Source: CAD feature listing. Evaluate the final solid. Frame: model axes, mm. A direction names the side the tool comes from. Give positions to 0.01 mm unless a question says otherwise; leave off trailing zeros. Order: outer loops, then holes, each group sorted by start corner. A loop starts at its lowest first (then second) coordinate and runs counter-clockwise, first axis right, second up.
1) Access query for faces 1 (the face through (2, -5, -2)), 2 (the face through (-2.003, 19.154, 0.631)), 3 (the face through (1.014, -3.768, 1.724)). Directions: +Z, -Z, +X, -X, +Y, -Y. A direction counts if a zero-diameter tool reaches every point of the face in a straight line with its end or side. Return the directions, or none.
2) Section A-A, the plane z = 0. Return loops of the section in (x, y).
3) Section B-B, the plane y = 10. Return loops of the section in (x, z), plus the area to 3 significant figures.
4) First-contact query: P1, Ø4, axis at x = -1.5, y = 1.5, coming from the -Z side; P2, Ø4, axis at y = 18.5, z = 1.5, coming from the -X side. Flat tips, straight axial feed; report the tip coordinate or a pass-through.
5) Draft query along Z for faces 4 (the face through (-2, -4, 0)), 5 (the face through (2.285, -2.268, 3.584)), 6 (the face through (0.99, -3.77, -1.74)), 7 (the face through (0, 30, 0)). Return one class per face: released by +Z, released by -Z, zero draft, split by the parting line, or undercut.
6) Material intervals for line 1 (Y direction, x = 2.5, z = -0.5); line 2 (Z direction, x = -1.5, y = 7), sorted ascending.
```python
from build123d import *

# Parameters (mm, degrees)
F0_R     = 4.25
F1_DEPTH = 5
F2_R     = 2.5
F3_DEPTH = 30
F4_R     = 2.5
F4_R_2   = 2.1
F5_DEPTH = 22
F7_DEPTH = 2.5
F8_SIZE  = 0.4


with BuildPart() as f1:
    # F0 (on Front) → F1 (new body)
    with BuildSketch(Plane.XZ):
        Circle(F0_R)
    extrude(amount=F1_DEPTH)

    # F2 (on face) → F3 (join)
    with BuildSketch(Plane(origin=(0, 0, 0), x_dir=(-1, 0, 0), z_dir=(0, 1, 0))):
        Circle(F2_R)
    extrude(amount=F3_DEPTH)

    # F4 (on face) → F5 (cut)
    with BuildSketch(Plane(origin=(0, 30, 0), x_dir=(-1, 0, 0), z_dir=(0, 1, 0))):
        Circle(F4_R)
        Circle(F4_R_2, mode=Mode.SUBTRACT)
    extrude(amount=-F5_DEPTH, mode=Mode.SUBTRACT)

    # F6 (on face) → F7 (cut)
    with BuildSketch(Plane.XZ.offset(5)):
        Polygon((0, -2.309401), (2, -1.154701), (2, 1.154701), (0, 2.309401), (-2, 1.154701), (-2, -1.154701), align=None)
    extrude(amount=-F7_DEPTH, mode=Mode.SUBTRACT)

    # F8
    f8_edges = [f1.edges().sort_by_distance(p)[0] for p in [
        (-4.25, -5, 0),
    ]]
    chamfer(f8_edges, length=F8_SIZE)


solid = f1.part
```
From the geometry:
1. face 1: +Z, -Z, +X, -X, -Y
1. face 2: +Y
1. face 3: -Y
2. outline: (-4.25, -4.6) - (-3.85, -5) - (-2, -5) - (-2, -2.5) - (2, -2.5) - (2, -5) - (3.85, -5) - (4.25, -4.6) - (4.25, 0) - (2.5, 0) - (2.5, 8) - (2.1, 8) - (2.1, 30) - (-2.1, 30) - (-2.1, 8) - (-2.5, 8) - (-2.5, 0) - (-4.25, 0) - close
3. outline: circle Ø4.2 at (0, 0)
3. area: 13.9 mm2
4. P1: stops at z = -4.25
4. P2: stops at x = -2.1
5. face 4: undercut
5. face 5: split by the parting line
5. face 6: undercut
5. face 7: zero draft
6. line 1: y = -5 to 0
6. line 2: z = -2 to 2
